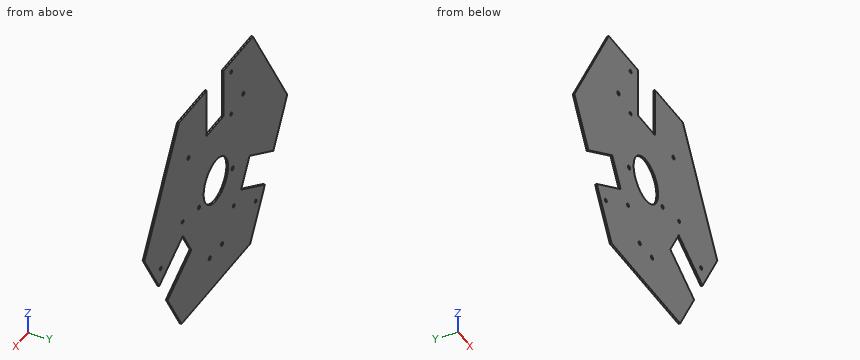
from build123d import *

# Parameters (mm, degrees)
SKETCH1_R           = 3
SKETCH1_R_2         = 3.5
SKETCH1_R_3         = 40
BOSS_EXTRUDE1_DEPTH = 3


with BuildPart() as part:
    # Sketch1 → Boss-Extrude1 (new body)
    with BuildSketch(Plane(origin=(0, 0, 0), x_dir=(1, 0, 0), z_dir=(0, 1, 0))):
        Polygon((158.205080757, 125.980762114), (112.5, 205.144284149), (-112.5, 205.144284149), (-160.705080757, 121.650635095), (-82.762794416, 76.650635095), (-95.262794416, 55), (-110.262794416, 29.019237886), (-188.205080757, 74.019237886), (-233.910161514, -5.144284149), (-121.410161514, -200), (-25, -200), (-25, -110), (0, -110), (30, -110), (30, -200), (121.410161514, -200), (233.910161514, -5.144284149), (185.705080757, 78.349364905), (107.762794416, 33.349364905), (80.262794416, 80.980762114), align=None)
        with Locations(Location((-50.14, -180, 0), (0, 0, 270))):
            Circle(SKETCH1_R, mode=Mode.SUBTRACT)
        with Locations(Location((-90, -108.599272381, 0), (0, 0, 270))):
            Circle(SKETCH1_R_2, mode=Mode.SUBTRACT)
        with Locations(Location((-50.14, -96.51, 0), (0, 0, 270))):
            Circle(SKETCH1_R, mode=Mode.SUBTRACT)
        with Locations(Location((90, -108.599272381, 0), (0, 0, 270))):
            Circle(SKETCH1_R_2, mode=Mode.SUBTRACT)
        with Locations(Location((0, 0, 0), (0, 0, 270))):
            Circle(SKETCH1_R_3, mode=Mode.SUBTRACT)
        with Locations(Location((-55, 14.522505884, 0), (0, 0, 270))):
            Circle(SKETCH1_R_2, mode=Mode.SUBTRACT)
        with Locations(Location((-58.510111719, 91.677513746, 0), (0, 0, 270))):
            Circle(SKETCH1_R, mode=Mode.SUBTRACT)
        with Locations(Location((-130.814572681, 133.422513746, 0), (0, 0, 270))):
            Circle(SKETCH1_R, mode=Mode.SUBTRACT)
        with Locations(Location((-20, 140.144284149, 0), (0, 0, 270))):
            Circle(SKETCH1_R_2, mode=Mode.SUBTRACT)
        with Locations(Location((55, 14.522505884, 0), (0, 0, 270))):
            Circle(SKETCH1_R_2, mode=Mode.SUBTRACT)
        with Locations(Location((108.953220611, 5.007486254, 0), (0, 0, 270))):
            Circle(SKETCH1_R, mode=Mode.SUBTRACT)
        with Locations(Location((180.954572681, 46.577486254, 0), (0, 0, 270))):
            Circle(SKETCH1_R, mode=Mode.SUBTRACT)
        with Locations(Location((20, 140.144284149, 0), (0, 0, 270))):
            Circle(SKETCH1_R_2, mode=Mode.SUBTRACT)
    extrude(amount=BOSS_EXTRUDE1_DEPTH)


solid = part.part
CAD build for the part. Positions are in the model's coordinates, mm. Round coordinates to 2 decimals unless told otherwise and drop trailing zeros. Write each loop counter-clockwise with the first axis right and the second up, starting at its lowest first coordinate (ties: lowest second). Pieces come first, ordered by that corner, then holes.
(1) Slice it at D-D, the plane x = 198. Write the cut outline in (y, z), and give its area (3 significant figures).
(2) Slice it at B-B, the plane y = 1.65. Count the separate pieces of the cut face and the enclosed holes in it, and give its area (3 significant figures).
(3) Probe line 1 along X through (y, z) = (1.65, 180); line 2 along X through (y, z) = (0.8, -48); line 3 along X through (y, z) = (2.3, -63.5). List the from-to ranges inside material, lowest first.
(4) Drop a flat-ended pin along its axis: P1, Ø9.5, axis at x = -58.51, z = -91.68, coming from the +Y side. Give the stop position or say it passes through.
(5) Slice it at A-A, the plane z = 121.5. Write the cut outline in (x, y), and give its area (3 significant figures).
(6) Slice it at C-C, the plane z = 52. Write the cut outline in (x, y), and give its area (3 significant figures).
From the geometry:
1. outline: (0, -57.05) - (3, -57.05) - (3, 67.34) - (0, 67.34) - close
1. area: 373 mm2
2. separate pieces: 1
2. enclosed holes: 13
2. area: 122,000 mm2
3. line 1: x = -132.96 to -53.14, -47.14 to -25, 30 to 132.96
3. line 2: x = -203.23 to -143.14, -99.3 to 99.3, 133.14 to 178.31, 183.6 to 203.23
3. line 3: x = -194.28 to -169.99, -90.36 to 90.36, 159.99 to 194.28
4. P1: stops at y = 3
5. outline: (-166.73, 0) - (-25, 0) - (-25, 3) - (-166.73, 3) - close; (30, 0) - (166.73, 0) - (166.73, 3) - (30, 3) - close
5. area: 835 mm2
6. outline: (-206.86, 0) - (206.86, 0) - (206.86, 3) - (-206.86, 3) - close
6. area: 1,240 mm2
